CAD build for the part. Positions are in the model's coordinates, mm. A direction names the side the tool comes from. Coordinates: 2 decimals unless noted, no trailing zeros. Write each loop counter-clockwise with the first axis right and the second up, starting at its lowest first coordinate (ties: lowest second). Pieces come first, ordered by that corner, then holes.
```python
from build123d import *

# Parameters (mm, degrees)
BASPROSKE_W         = 7
BASPROSKE_H         = 13.5
TOOTHCUT_DEPTH      = 21.334699408
TEETHCUTS_COUNT     = 25
TEETHCUTS_ANGLE     = 345.6
BORSKE_R            = 0.4
BORE_DEPTH          = 50.0000508
SKETCH_1_R          = 1.65
CUT_EXTRUDE_1_DEPTH = 10
SKETCH_2_W          = 30
SKETCH_2_H          = 10
SKETCH_2_R          = 1.65
EXTRUDE_2_DEPTH     = 5
CUT_EXTRUDE_2_DEPTH = 2.5


with BuildPart() as part:
    # BasProSke → Base-Revolve (revolve)
    with BuildSketch(Plane(origin=(0, 0, 0), x_dir=(1, 0, 0), z_dir=(0, 1, 0)), mode=Mode.PRIVATE) as base_revolve_sk:
        with Locations((3.5, 6.75)):
            Rectangle(BASPROSKE_W, BASPROSKE_H)
    revolve(base_revolve_sk.sketch.rotate(Axis((-10, 0, 0), (1, 0, 0)), 180), axis=Axis((-10, 0, 0), (1, 0, 0)))

    # TooCutSke → ToothCut (cut, through all)
    with BuildSketch(Plane(origin=(0, 0, 0), x_dir=(0, 0, -1), z_dir=(1, 0, 0))):
        with BuildLine():
            ThreePointArc((0.480087995, 11.238750665), (0, 11.249), (-0.480087995, 11.238750665))
            ThreePointArc((-0.480087995, 11.238750665), (-0.821124963, 12.40220054), (-1.432168974, 13.449361962))
            ThreePointArc((-1.432168974, 13.449361962), (0, 13.5254), (1.432168974, 13.449361962))
            ThreePointArc((1.432168974, 13.449361962), (0.821124963, 12.40220054), (0.480087995, 11.238750665))
        make_face()
    toothcut = extrude(amount=TOOTHCUT_DEPTH, mode=Mode.SUBTRACT)

    # TeethCuts: ToothCut ×25 about axis
    teethcuts_axis = Axis((-10, 0, 0), (1, 0, 0))
    for i in range(1, TEETHCUTS_COUNT):
        add(toothcut.rotate(teethcuts_axis, i * TEETHCUTS_ANGLE / (TEETHCUTS_COUNT - 1)), mode=Mode.SUBTRACT)

    # BorSke → Bore (cut, symmetric)
    with BuildSketch(Plane(origin=(0, 0, 0), x_dir=(0, 0, -1), z_dir=(1, 0, 0))):
        with Locations(Location((0, 0, 0), (0, 0, 180))):
            Circle(BORSKE_R)
    extrude(amount=BORE_DEPTH, both=True, mode=Mode.SUBTRACT)

    # 草图1 → 切除-拉伸1 (cut)
    with BuildSketch(Plane(origin=(7, 0, 0), x_dir=(0, 0, -1), z_dir=(1, 0, 0))):
        Circle(SKETCH_1_R)
    extrude(amount=-CUT_EXTRUDE_1_DEPTH, mode=Mode.SUBTRACT)

    # 草图2 → 凸台-拉伸2 (add)
    with BuildSketch(Plane(origin=(7, 0, 0), x_dir=(0, 0, -1), z_dir=(1, 0, 0))):
        with Locations((-24, 0)):
            Rectangle(SKETCH_2_W, SKETCH_2_H)
        with Locations((-31, 0)):
            Circle(SKETCH_2_R, mode=Mode.SUBTRACT)
        with Locations((-19, 0)):
            Circle(SKETCH_2_R, mode=Mode.SUBTRACT)
    extrude(amount=-EXTRUDE_2_DEPTH)

    # 草图3 → 切除-拉伸2 (cut)
    with BuildSketch(Plane(origin=(7, 0, 0), x_dir=(0, 0, -1), z_dir=(1, 0, 0))):
        Polygon((-27.651368439, 0), (-29.325684219, 2.9), (-32.674315781, 2.9), (-34.348631561, 0), (-32.674315781, -2.9), (-29.325684219, -2.9), align=None)
        Polygon((-15.651368439, 0), (-17.325684219, 2.9), (-20.674315781, 2.9), (-22.348631561, 0), (-20.674315781, -2.9), (-17.325684219, -2.9), align=None)
    extrude(amount=-CUT_EXTRUDE_2_DEPTH, mode=Mode.SUBTRACT)


solid = part.part
```
Item 1: Saw through at A-A, the plane z = 19. Write the cut outline in (x, y), and give its area (4 significant figures).
Item 2: Which spindle directions (+Z, -Z, +X, -X, +Y, -Y) get a long thin tool onto all of the face, cutting with end or side? Do faces 1 (the cylindrical face through (3.451, 4.593, -11.518)), 2 (the cylindrical face through (3.45, -10.49, 6.62)), 3 (the flat face through (5.768, -1.43, 33.523)), 4 (the cylindrical face through (0.986, 0.713, 11.226)). Say none if no direction does.
Item 3: Flat gauge pins, fed straight in: pin 1 Ø4 at (x, z) = (6, 28) entering from +Y; pin 2 Ø2 at (x, y) = (5.5, 8) entering from -Z; pin 3 Ø6.5 at (y, z) = (0.5, 18.5) entering from +X; pin 4 Ø4 at (y, z) = (3.5, 28) entering from -X. Where does each tip first touch, or does it go through?
Item 4: Two-plate mould, pull along Y, no slides. Class faces 5 (the cylindrical face through (3.45, -12.2, 2.37)), 6 (the cylindrical face through (3.45, 11.78, 3.86)), 7 (the flat face through (4.5, 1.3, 29.6)): +Y half, -Y half, draft (parallel to the pull), parting line (faces both ways), or undercut.
Item 5: Wall check: line 1 along Y through (x, z) = (2.95, 19); line 2 along Z through (x, y) = (6.75, 11.5); line 3 along Z through (x, y) = (6.25, -9.75). Give the ranges that are in metal, low to high.
Item 6: Saw through at B-B, the plane x = 5.5. State how many separate pieces and enclosed holes the cut face has, and give its area (3 significant figures).
Item 7: Saw through at C-C, the plane y = -6.25. Write the cut outline in (x, z), and give its area (3 significant figures).
Working result:
1. outline: (2, -5) - (7, -5) - (7, -2.9) - (4.5, -2.9) - (4.5, -1.65) - (2, -1.65) - close; (2, 1.65) - (4.5, 1.65) - (4.5, 2.9) - (7, 2.9) - (7, 5) - (2, 5) - close
1. area: 27.25 mm2
2. face 1: -Z, +X, -X
2. face 2: +X, -X
2. face 3: +X
2. face 4: +Z, -X
3. pin 1: stops at y = 5
3. pin 2: stops at z = -10.58
3. pin 3: stops at x = 7
3. pin 4: stops at x = 2
4. face 5: -Y half
4. face 6: +Y half
4. face 7: undercut
5. line 1: y = -5 to -1.65, 1.65 to 5
5. line 2: z = -5.27 to -3.66, -2.35 to -0.53, 0.53 to 2.35, 3.66 to 5.27
5. line 3: z = -9.34 to -8.32, -6.39 to 6.39, 8.32 to 9.34
6. separate pieces: 1
6. enclosed holes: 3
6. area: 681 mm2
7. outline: (0, -11.06) - (7, -11.06) - (7, 11.06) - (0, 11.06) - close
7. area: 155 mm2
